from build123d import *

# Parameters (mm, degrees)
SKETCH3_R           = 8.05
BOSS_EXTRUDE1_DEPTH = 30
SKETCH4_R           = 8.05
SKETCH4_R_2         = 4.3
BOSS_EXTRUDE2_DEPTH = 25
CHAMFER1_SIZE       = 3
FILLET1_R           = 11
SKETCH5_R           = 1.65
CUT_EXTRUDE1_DEPTH  = 81.777378375
SKETCH6_R           = 3
CUT_EXTRUDE2_DEPTH  = 3
SKETCH7_W           = 22
SKETCH7_H           = 18.6
CUT_EXTRUDE3_DEPTH  = 88.398998033
FILLET2_R           = 2
SKETCH8_R           = 1.65
CUT_EXTRUDE4_DEPTH  = 73.43358938
CUT_EXTRUDE5_DEPTH  = 73.43358938
FILLET3_R           = 5
SKETCH10_R          = 3
CUT_EXTRUDE6_DEPTH  = 3
CUT_EXTRUDE7_DEPTH  = 73.43358938
SKETCH12_R          = 2.1
CUT_EXTRUDE8_DEPTH  = 5


# Some blends are built 0.0001 mm under size
with BuildPart() as part:
    # Sketch3 → Boss-Extrude1 (new body)
    with BuildSketch(Plane.XY):
        with BuildLine():
            Line((-25.5, 0), (-36.354158733, 0))
            Line((-36.354158733, 0), (-36.354158733, -8))
            Line((-36.354158733, -8), (-27.354158733, -8))
            ThreePointArc((-27.354158733, -8), (-21.246325292, -18.995885385), (-11, -26.29163365))
            Line((-11, -26.29163365), (-11, -73.6))
            Line((-11, -73.6), (11, -73.6))
            Line((11, -73.6), (11, -26.29163365))
            ThreePointArc((11, -26.29163365), (21.246325292, -18.995885385), (27.354158733, -8))
            Line((27.354158733, -8), (36.354158733, -8))
            Line((36.354158733, -8), (36.354158733, 0))
            Line((36.354158733, 0), (25.5, 0))
            ThreePointArc((25.5, 0), (0, -25.5), (-25.5, 0))
        make_face()
        with Locations((0, -62.6)):
            Circle(SKETCH3_R, mode=Mode.SUBTRACT)
    extrude(amount=BOSS_EXTRUDE1_DEPTH)

    # Sketch4 → Boss-Extrude2 (add)
    with BuildSketch(Plane.XY):
        with Locations(Location((0, -62.6, 0), (0, 0, 180))):
            Circle(SKETCH4_R)
        with Locations(Location((0, -62.6, 0), (0, 0, 180))):
            Circle(SKETCH4_R_2, mode=Mode.SUBTRACT)
    extrude(amount=BOSS_EXTRUDE2_DEPTH)

    # Chamfer1
    chamfer1_edges = [part.edges().sort_by_distance(p)[0] for p in [
        (0, -73.6, 0),
    ]]
    chamfer(chamfer1_edges, length=CHAMFER1_SIZE)

    # Fillet1
    fillet1_edges = [part.edges().sort_by_distance(p)[0] for p in [
        (-11, -73.6, 16.5),
        (11, -73.6, 16.5),
    ]]
    fillet(fillet1_edges, radius=FILLET1_R - 0.0001)  # a hair under: the kernel refuses the full size

    # Sketch5 → Cut-Extrude1 (cut, through all)
    with BuildSketch(Plane.XZ.offset(8)):
        with Locations((31.854158733, 15)):
            Circle(SKETCH5_R)
    cut_extrude1 = extrude(amount=-CUT_EXTRUDE1_DEPTH, mode=Mode.SUBTRACT)

    # Sketch6 → Cut-Extrude2 (cut)
    with BuildSketch(Plane.XZ.offset(8)):
        with Locations((31.854158733, 15)):
            Circle(SKETCH6_R)
    cut_extrude2 = extrude(amount=-CUT_EXTRUDE2_DEPTH, mode=Mode.SUBTRACT)

    # Mirror1: Cut-Extrude1, Cut-Extrude2 across plane
    add(cut_extrude1.mirror(Plane(origin=(0, 0, 0), x_dir=(0, 0, 1), z_dir=(1, 0, 0))), mode=Mode.SUBTRACT)
    add(cut_extrude2.mirror(Plane(origin=(0, 0, 0), x_dir=(0, 0, 1), z_dir=(1, 0, 0))), mode=Mode.SUBTRACT)

    # Sketch7 → Cut-Extrude3 (cut, through all)
    with BuildSketch(Plane.XY.offset(30)):
        with Locations((0, -64.3)):
            Rectangle(SKETCH7_W, SKETCH7_H)
    extrude(amount=-CUT_EXTRUDE3_DEPTH, mode=Mode.SUBTRACT)

    # Fillet2
    # the kernel refuses this fillet: 2 mm, written as the material it adds along each edge
    with BuildSketch(Plane(origin=(27.354158733, -8, 0), x_dir=(1, 0, 0), z_dir=(0, 0, 1))) as fillet2_piece_1:
        with BuildLine():
            CenterArc((1.459900335, -2), FILLET2_R, 90, 70.860525549)
            ThreePointArc((-0.429546161, -1.344262295), (-0.206451392, -0.674790264), (0, 0))
            Line((0, 0), (1.459900335, 0))
        make_face()
    extrude(amount=30)
    with BuildSketch(Plane(origin=(-27.354158733, -8, 0), x_dir=(0.30437860573795156, -0.9525511347791366, 0), z_dir=(0, 0, 1))) as fillet2_piece_2:
        with BuildLine():
            CenterArc((1.460739841, -1.999386932), FILLET2_R, 91.418691197, 70.860525549)
            Line((-0.444362429, -1.390629721), (0, 0))
            ThreePointArc((0, 0), (0.705611618, -0.008736212), (1.411223236, 0))
        make_face()
    extrude(amount=30)
    # the kernel refuses this fillet: 2 mm, written as the material it takes off along each edge
    with BuildSketch(Plane(origin=(-36.354158733, 0, -5), x_dir=(0, -1, 0), z_dir=(0, 0, 1)), Plane(origin=(36.354158733, 0, -5), x_dir=(-1, 0, 0), z_dir=(0, 0, 1)), Plane(origin=(36.354158733, -8, -5), x_dir=(0, 1, 0), z_dir=(0, 0, 1)), Plane(origin=(-36.354158733, -8, -5), x_dir=(1, 0, 0), z_dir=(0, 0, 1))) as fillet2_2_piece_1:
        with BuildLine():
            CenterArc((FILLET2_R, FILLET2_R), FILLET2_R, 180, 90)
            Line((0, FILLET2_R), (0, 0))
            Line((0, 0), (FILLET2_R, 0))
        make_face()
    extrude(amount=40, mode=Mode.SUBTRACT)
    with BuildSketch(Plane(origin=(-25.5, 0, -4.81794076), x_dir=(-1, 0, 0), z_dir=(0, 0, 1))) as fillet2_2_piece_2:
        with BuildLine():
            CenterArc((1.927176304, 2), FILLET2_R, 184.170647912, 85.829352088)
            ThreePointArc((-0.067527427, 1.854545455), (-0.016887449, 0.927887223), (0, 0))
            Line((0, 0), (1.927176304, 0))
        make_face()
    extrude(amount=39.635881519, mode=Mode.SUBTRACT)
    with BuildSketch(Plane(origin=(25.5, 0, -4.81794076), x_dir=(-0.03638773424584517, -0.9993377471087809, 0), z_dir=(0, 0, 1))) as fillet2_2_piece_3:
        with BuildLine():
            CenterArc((1.928549915, 1.998675494), FILLET2_R, 182.085323956, 85.829352088)
            Line((-0.070125579, 1.925900026), (0, 0))
            ThreePointArc((0, 0), (0.927887223, 0.016887449), (1.855774447, 0))
        make_face()
    extrude(amount=39.635881519, mode=Mode.SUBTRACT)

    # Sketch8 → Cut-Extrude4 (cut, through all)
    with BuildSketch(Plane.XY.offset(30)):
        with Locations((4.5, -49)):
            Circle(SKETCH8_R)
        with Locations((-4.5, -49)):
            Circle(SKETCH8_R)
    extrude(amount=-CUT_EXTRUDE4_DEPTH, mode=Mode.SUBTRACT)

    # Sketch9 → Cut-Extrude5 (cut, through all)
    with BuildSketch(Plane.XY.offset(30)):
        with BuildLine():
            Line((-8.75, -55), (-8.75, -27.12355987))
            ThreePointArc((-8.75, -27.12355987), (-9.883756892, -26.73128036), (-11, -26.29163365))
            Line((-11, -26.29163365), (-11, -55))
            Line((-11, -55), (-8.75, -55))
        make_face()
        with BuildLine():
            Line((8.75, -55), (8.75, -27.12355987))
            ThreePointArc((8.75, -27.12355987), (9.883756892, -26.73128036), (11, -26.29163365))
            Line((11, -26.29163365), (11, -55))
            Line((11, -55), (8.75, -55))
        make_face()
    extrude(amount=-CUT_EXTRUDE5_DEPTH, mode=Mode.SUBTRACT)

    # Fillet3
    fillet3_edges = [part.edges().sort_by_distance(p)[0] for p in [
        (-8.75, -55, 15),
        (-8.75, -27.12355987, 15),
        (8.75, -55, 15),
        (8.75, -27.12355987, 15),
    ]]
    fillet(fillet3_edges, radius=FILLET3_R)

    # Sketch10 → Cut-Extrude6 (cut)
    with BuildSketch(Plane.XY.offset(30)):
        with Locations((4.5, -49)):
            Circle(SKETCH10_R)
        with Locations((-4.5, -49)):
            Circle(SKETCH10_R)
    extrude(amount=-CUT_EXTRUDE6_DEPTH, mode=Mode.SUBTRACT)

    # Sketch11 → Cut-Extrude7 (cut, through all)
    with BuildSketch(Plane.XY.offset(30)):
        with BuildLine():
            Line((8.75, -30.548117782), (8.75, -50))
            ThreePointArc((8.75, -50), (7.285533906, -53.535533906), (3.75, -55))
            Line((3.75, -55), (-3.75, -55))
            ThreePointArc((-3.75, -55), (-7.285533906, -53.535533906), (-8.75, -50))
            Line((-8.75, -50), (-8.75, -30.548117782))
            ThreePointArc((-8.75, -30.548117782), (-8.031860325, -32.281860325), (-6.298117782, -33))
            Line((-6.298117782, -33), (6.298117782, -33))
            ThreePointArc((6.298117782, -33), (8.031860325, -32.281860325), (8.75, -30.548117782))
        make_face()
    extrude(amount=-CUT_EXTRUDE7_DEPTH, mode=Mode.SUBTRACT)

    # Sketch12 → Cut-Extrude8 (cut)
    with BuildSketch(Plane.XZ.offset(33)):
        with Locations(Location((-4.5, 15, 0), (0, 0, 270))):
            Circle(SKETCH12_R)
        with Locations(Location((4.5, 15, 0), (0, 0, 270))):
            Circle(SKETCH12_R)
    extrude(amount=-CUT_EXTRUDE8_DEPTH, mode=Mode.SUBTRACT)


solid = part.part
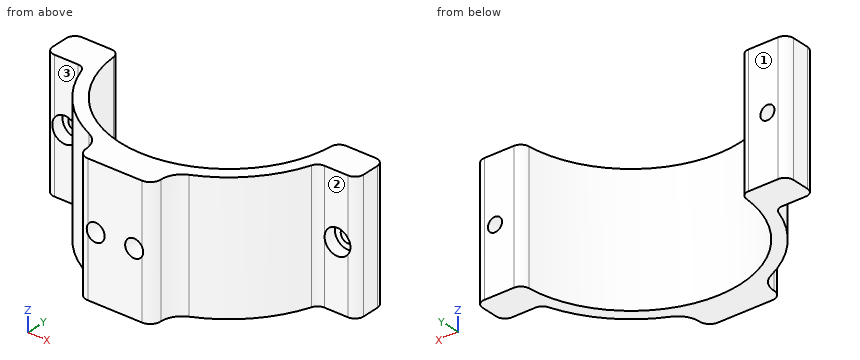
Input: part model. Units: mm. Frame: model coordinates. Face numbers are marked on the shaded views. A direction names the side the tool comes from. Give positions to 0.01 mm unless a question says otherwise; leave off trailing zeros. Write each loop counter-clockwise with the first axis right and the second up, starting at its lowest first coordinate (ties: lowest second). Pieces come first, ordered by that corner, then holes. Notation, with made-up numbers: M 23.5,30.5 L 73.5,30.5 A21 ccw 73.5,55.5 Z; hole C 0,85.25 d8. An arc over 180 degrees is marked long. Write item = value, one per line. Start each with the question number.
1) Cut plane D-D on y = -21.5. Return the cut outline in (x, z), then the cut area to 3 significant figures.
2) Material intervals for line 1 along Z through (x, y) = (-4.5, -31.65); line 2 along Y through (x, z) = (29, 23); line 3 along X through (y, z) = (-7.2, 15), sorted ascending. Write a range as [from, to].
3) First-contact query: pin 1 Ø4.5 at (x, z) = (-4, 16) entering from -Y; pin 2 Ø8 at (x, z) = (-31.85, 15) entering from -Y; pin 3 Ø8 at (y, z) = (-11.5, 12.5) entering from -X; pin 4 Ø6.5 at (x, z) = (-33, 14.5) entering from -Y. Flat tips, straight axial feed; report the tip coordinate or a pass-through.
4) Cut plane C-C on x = 0. Return the cut outline in (y, z), then the cut area to 3 significant figures.
5) Cut plane A-A on x = 31. Return the cut outline in (y, z), then the cut area to 3 significant figures.
6) Cut plane B-B on y = -12. Return the cut outline in (x, z), then the cut area to 3 significant figures.
7) Reachability of the marked faces 1, 2 and 3 from +Z, -Z, +X, -X, +Y, -Y: full face, straight path, thin tool, end or side. Return the list, or none.
Solved:
q1.outline = M -18.71,0 L -13.71,0 L -13.71,30 L -18.71,30 Z; M 13.71,0 L 18.71,0 L 18.71,30 L 13.71,30 Z
q1.area = 300 mm2
q2.line_1 = [0, 12.9], [17.1, 30]
q2.line_2 = [-8, 0]
q2.line_3 = [-35.95, -34.85], [-28.85, -24.46], [24.46, 28.85], [34.85, 35.95]
q3.pin_1 = -33
q3.pin_2 = -8.25
q3.pin_3 = -35.68
q3.pin_4 = -8
q4.outline = M -33,0 L -25.5,0 L -25.5,30 L -33,30 Z
q4.area = 225 mm2
q5.outline = M -8,0 L 0,0 L 0,13.59 L -5,13.59 L -5,12.12 L -8,12.12 Z; M -8,17.88 L -5,17.88 L -5,16.41 L 0,16.41 L 0,30 L -8,30 Z
q5.area = 209 mm2
q6.outline = M -25.85,0 L -22.5,0 L -22.5,30 L -25.85,30 Z; M 22.5,0 L 25.85,0 L 25.85,30 L 22.5,30 Z
q6.area = 201 mm2
q7.face_1 = +Z, -Z, +X, -X, +Y
q7.face_2 = +Z, -Z, +X, -Y
q7.face_3 = +Z, -Z, -X, -Y
